Autodesk Inventor part; units mm, degrees
ref_plane "YZ Plane" through (0, 0, 0) normal (1, 0, 0) x (0, 1, 0)
ref_plane "XZ Plane" through (0, 0, 0) normal (0, 1, 0) x (-1, 0, 0)
ref_plane "XY Plane" through (0, 0, 0) normal (0, 0, 1) x (1, 0, 0)
sketch "Sketch1" plane through (0, 0, 0) normal (0, 0, 1) x (1, 0, 0)
  circle A0 centre (0, 0) radius 7
  circle A1 centre (52.2854, 37.1495) radius 7
  circle A2 centre (3.2487, 67.4218) radius 7
  circle A3 centre (73.2479, 48.3549) radius 2.15
  circle A4 centre (73.9366, 30.5749) radius 3.15 construction
  circle A5 centre (58.8599, 58.8007) radius 3.15 construction
  circle A6 centre (4.7755, 90.6548) radius 2.15
  circle A7 centre (-59.4554, -13.318) radius 2.15
  circle A8 centre (9.0171, -55.618) radius 2.15
  circle A9 centre (38.0853, -27.4589) radius 3.15 construction
  circle A10 centre (-27.4589, -38.0853) radius 3.5 construction
  line L0 (38.0853, -27.4589) -> (9.0171, -55.618) construction
  line L1 (9.0171, -55.618) -> (-27.4589, -38.0853) construction
  line L2 (9.0171, -55.618) -> (73.2479, 48.3549)
  line L3 (92.2333, 46.5881) -> (17.5545, -74.2973) construction
  line L4 (-27.4589, -38.0853) -> (-59.4554, -13.318) construction
  line L5 (-59.4554, -13.318) -> (-42.6755, 23.5008) construction
  line L6 (-59.4554, -13.318) -> (4.7755, 90.6548)
  line L7 (4.7755, 90.6548) -> (73.2479, 48.3549)
  line L8 (9.0171, -55.618) -> (-59.4554, -13.318)
  circle A11 centre (9.0171, -55.618) radius 6
  circle A12 centre (-59.4554, -13.318) radius 6
  circle A13 centre (4.7755, 90.6548) radius 6
  circle A14 centre (73.2479, 48.3549) radius 6
  point P0 (0, 0)
  point P1 (3.9125, -52.4646)
  point P2 (12.1704, -50.5134)
  point P3 (70.0945, 43.2504)
  point P4 (68.1434, 51.5083)
  point P5 (9.88, 87.5015)
  point P6 (1.6221, 85.5503)
  point P7 (-56.302, -8.2135)
  point P8 (-54.3509, -16.4714)
  point P9 (71.4188, 49.4849)
  point P10 (72.118, 46.5258)
  point P11 (3.6455, 88.8257)
  point P12 (6.6046, 89.5249)
  point P13 (-57.6263, -14.448)
  point P14 (-58.3254, -11.4889)
  point P15 (10.147, -53.7888)
  point P16 (7.1879, -54.488)
  dimension "d0" = 4.3
  dimension "d1" = 17.78
  dimension "d2" = 17.78
  dimension "d3" = 4.3
  dimension "d4" = 4.3
  dimension "d5" = 4.3
  dimension "d6" = 40.4622
  dimension "d7" = 12
  dimension "d8" = 12
  dimension "d9" = 12
  dimension "d10" = 12
extrude "Extrusion1" add sketch "Sketch1" along normal blind 3.175 contours A3 L7 A14 L2 | A3 L2 A14 L7 | A14 L2 A11 L8 A12 L6 A13 L7 | A13 L6 A6 L7 | L7 A6 L6 A13 | A11 L8 A8 L2 | L2 A8 L8 A11 | A12 L8 A7 L6 | L6 A7 L8 A12
fillet "Fillet1" radius 3.175 8 edges at (3.9125, -52.4646, 1.5875) (-54.3509, -16.4714, 1.5875) (-56.302, -8.2135, 1.5875) (1.6221, 85.5503, 1.5875) (9.88, 87.5015, 1.5875) (68.1434, 51.5083, 1.5875) (70.0945, 43.2504, 1.5875) (12.1704, -50.5134, 1.5875)
sketch "Sketch2" plane through (0, 0, 0) normal (0, 0, -1) x (-1, 0, 0)
  arc A0 (-13.742, -51.92) -> (-13.5412, -48.2946) centre (-16.2423, -49.9632) ccw
  line L0 (-13.5412, -48.2946) -> (-68.7238, 41.0315)
  arc A1 (-68.7238, 41.0315) -> (-72.0558, 42.4746) centre (-71.4249, 39.3629) ccw
  arc A2 (-69.55, 53.0799) -> (-72.0558, 42.4746) centre (-73.2479, 48.3549) ccw
  arc A3 (-69.55, 53.0799) -> (-65.9245, 52.8791) centre (-67.5932, 55.5802) ccw
  line L1 (-65.9245, 52.8791) -> (-12.0989, 86.1307)
  arc A4 (-12.0989, 86.1307) -> (-10.6559, 89.4627) centre (-13.7676, 88.8318) ccw
  arc A5 (-0.0505, 86.9569) -> (-10.6559, 89.4627) centre (-4.7755, 90.6548) ccw
  arc A6 (-0.0505, 86.9569) -> (-0.2513, 83.3315) centre (2.4498, 85.0001) ccw
  line L2 (-0.2513, 83.3315) -> (54.9312, -5.9946)
  arc A7 (54.9312, -5.9946) -> (58.2632, -7.4377) centre (57.6324, -4.326) ccw
  arc A8 (55.7575, -18.043) -> (58.2632, -7.4377) centre (59.4554, -13.318) ccw
  arc A9 (55.7575, -18.043) -> (52.132, -17.8422) centre (53.8007, -20.5433) ccw
  line L3 (52.132, -17.8422) -> (-1.6937, -51.0938)
  arc A10 (-1.6937, -51.0938) -> (-3.1367, -54.4258) centre (-0.025, -53.795) ccw
  arc A11 (-13.742, -51.92) -> (-3.1367, -54.4258) centre (-9.0171, -55.618) ccw
  circle A12 centre (-73.2479, 48.3549) radius 2.15
  circle A13 centre (0, 0) radius 7
  circle A14 centre (-52.2854, 37.1495) radius 7
  circle A15 centre (-3.2487, 67.4218) radius 7
  circle A16 centre (-4.7755, 90.6548) radius 2.15
  circle A17 centre (59.4554, -13.318) radius 2.15
  circle A18 centre (-9.0171, -55.618) radius 2.15
  line L4 (-50.3461, 20.9487) -> (-14.2871, -37.4213)
  arc A19 (-9.7416, -55.0509) -> (-9.2194, -45.6247) centre (-16.2423, -49.9632) ccw
  arc A20 (-9.7416, -55.0509) -> (-8.1154, -55.4352) centre (-9.0171, -55.618) ccw
  arc A21 (-4.3635, -46.772) -> (-8.1154, -55.4352) centre (-0.025, -53.795) ccw
  line L5 (0.8339, -43.5612) -> (42.6394, -17.7352)
  arc A22 (58.8884, -14.0425) -> (49.4621, -13.5204) centre (53.8007, -20.5433) ccw
  arc A23 (58.8884, -14.0425) -> (59.2726, -12.4164) centre (59.4554, -13.318) ccw
  arc A24 (50.6094, -8.6645) -> (59.2726, -12.4164) centre (57.6324, -4.326) ccw
  line L6 (46.6959, -2.3296) -> (9.6075, 57.7068)
  arc A25 (-4.051, 90.0878) -> (-4.5732, 80.6616) centre (2.4498, 85.0001) ccw
  arc A26 (-4.051, 90.0878) -> (-5.6771, 90.4721) centre (-4.7755, 90.6548) ccw
  arc A27 (-9.429, 81.8089) -> (-5.6771, 90.4721) centre (-13.7676, 88.8318) ccw
  line L7 (-11.3353, 80.6312) -> (-60.8723, 50.029)
  arc A28 (-72.6809, 49.0794) -> (-63.2547, 48.5572) centre (-67.5932, 55.5802) ccw
  arc A29 (-72.6809, 49.0794) -> (-73.0651, 47.4533) centre (-73.2479, 48.3549) ccw
  arc A30 (-64.402, 43.7014) -> (-73.0651, 47.4533) centre (-71.4249, 39.3629) ccw
  line L8 (-9.0171, -55.618) -> (0, 0) construction
  line L9 (0, 0) -> (59.4554, -13.318) construction
  line L10 (0, 0) -> (-3.2487, 67.4218) construction
  line L11 (-3.2487, 67.4218) -> (-4.7755, 90.6548) construction
  line L12 (0, 0) -> (-52.2854, 37.1495) construction
  line L13 (-52.2854, 37.1495) -> (-73.2479, 48.3549) construction
  line L14 (-52.2854, 37.1495) -> (-3.2487, 67.4218) construction
  line L15 (-4.7708, -13.5552) -> (-8.4519, -36.2607)
  line L16 (-11.5243, -55.2115) -> (-6.5098, -56.0245) construction
  line L17 (-3.9689, -40.352) -> (0.2437, -14.3682)
  line L18 (2.5073, -0.4065) -> (-2.5073, 0.4065) construction
  line L19 (-2.5073, 0.4065) -> (-6.5098, -56.0245) construction
  line L20 (-11.5243, -55.2115) -> (2.5073, -0.4065) construction
  line L21 (-39.2842, 31.0278) -> (-10.0588, 10.2628)
  line L22 (1.4712, 2.0706) -> (-1.4712, -2.0706) construction
  line L23 (-13.0012, 6.1217) -> (-42.2265, 26.8867)
  line L24 (-53.7566, 35.0789) -> (-50.8142, 39.2201) construction
  line L25 (-50.8142, 39.2201) -> (-1.4712, -2.0706) construction
  line L26 (1.4712, 2.0706) -> (-53.7566, 35.0789) construction
  line L27 (14.3572, -0.6131) -> (43.3008, -7.0964)
  line L28 (60.0106, -10.8395) -> (58.9002, -15.7966) construction
  line L29 (41.6647, -11.9359) -> (13.2468, -5.5702)
  line L30 (-0.5552, -2.4786) -> (0.5552, 2.4786) construction
  line L31 (0.5552, 2.4786) -> (58.9002, -15.7966) construction
  line L32 (60.0106, -10.8395) -> (-0.5552, -2.4786) construction
  line L33 (-3.2178, 14.0054) -> (-5.1051, 53.1719)
  line L34 (-5.7858, 67.2995) -> (-0.7117, 67.544) construction
  line L35 (-0.0309, 53.4164) -> (1.8563, 14.2499)
  line L36 (2.5371, 0.1222) -> (-2.5371, -0.1222) construction
  line L37 (-2.5371, -0.1222) -> (-0.7117, 67.544) construction
  line L38 (-5.7858, 67.2995) -> (2.5371, 0.1222) construction
  line L39 (-13.9498, 57.8305) -> (-38.9157, 42.4181)
  line L40 (-50.9511, 34.9882) -> (-53.6197, 39.3108) construction
  line L41 (-41.5843, 46.7407) -> (-16.6184, 62.1532)
  line L42 (-4.583, 69.5831) -> (-1.9145, 65.2604) construction
  line L43 (-1.9145, 65.2604) -> (-53.6197, 39.3108) construction
  line L44 (-50.9511, 34.9882) -> (-4.583, 69.5831) construction
  line L45 (-63.5617, 46.0573) -> (-60.7004, 44.5278)
  line L46 (-72.0505, 50.595) -> (-74.4453, 46.1149) construction
  line L47 (-74.4453, 46.1149) -> (-53.4828, 34.9094)
  line L48 (-53.4828, 34.9094) -> (-51.088, 39.3895) construction
  line L49 (-51.088, 39.3895) -> (-74.4453, 46.1149) construction
  line L50 (-72.0505, 50.595) -> (-53.4828, 34.9094) construction
  line L51 (-2.241, 90.8214) -> (-0.7142, 67.5883) construction
  line L52 (-0.7142, 67.5883) -> (-5.7833, 67.2552) construction
  line L53 (-6.7107, 81.3688) -> (-6.4984, 78.1383) construction
  line L54 (-7.31, 90.4883) -> (-2.241, 90.8214) construction
  line L55 (-2.241, 90.8214) -> (-5.7833, 67.2552) construction
  line L56 (-0.7142, 67.5883) -> (-7.31, 90.4883) construction
  arc A31 (-3.9689, -40.352) -> (0.8339, -43.5612) centre (-0.8348, -40.8601) ccw
  arc A32 (-14.2871, -37.4213) -> (-8.4519, -36.2607) centre (-11.586, -35.7526) ccw
  arc A33 (42.6394, -17.7352) -> (41.6647, -11.9359) centre (40.9707, -15.0341) ccw
  arc A34 (43.3008, -7.0964) -> (46.6959, -2.3296) centre (43.9948, -3.9982) ccw
  arc A35 (-5.1051, 53.1719) -> (-7.23, 56.0167) centre (-8.2764, 53.0191) ccw
  arc A36 (-8.499, 78.3012) -> (-6.7107, 81.3688) centre (-9.8789, 81.1606) ccw
  arc A37 (-8.499, 78.3012) -> (-15.1565, 65.3891) centre (-3.2487, 67.4218) ccw
  arc A38 (-10.4019, 57.6874) -> (-7.23, 56.0167) centre (-3.2487, 67.4218) ccw
  arc A39 (-10.4019, 57.6874) -> (-13.9498, 57.8305) centre (-12.282, 55.1289) ccw
  arc A40 (-16.6184, 62.1532) -> (-15.1565, 65.3891) centre (-18.2862, 64.8548) ccw
  arc A41 (-6.4984, 78.1383) -> (-11.3353, 80.6312) centre (-9.6666, 77.9301) ccw
  arc A42 (-40.5339, 34.3515) -> (-40.3776, 39.1822) centre (-52.2854, 37.1495) ccw
  arc A43 (-42.2265, 26.8867) -> (-45.7763, 26.9731) centre (-44.0655, 24.2985) ccw
  arc A44 (-45.1322, 46.8839) -> (-60.0296, 46.4206) centre (-52.2854, 37.1495) ccw
  arc A45 (-48.6108, 25.6419) -> (-45.7763, 26.9731) centre (-52.2854, 37.1495) ccw
  arc A46 (-48.6108, 25.6419) -> (-50.3461, 20.9487) centre (-47.645, 22.6174) ccw
  arc A47 (-45.1322, 46.8839) -> (-41.5843, 46.7407) centre (-43.2521, 49.4424) ccw
  arc A48 (-63.5617, 46.0573) -> (-60.0296, 46.4206) centre (-62.065, 48.8574) ccw
  arc A49 (-60.8723, 50.029) -> (-60.7004, 44.5278) centre (-59.2036, 47.3279) ccw
  arc A50 (-40.5339, 34.3515) -> (-39.2842, 31.0278) centre (-37.4452, 33.616) ccw
  arc A51 (-38.9157, 42.4181) -> (-40.3776, 39.1822) centre (-37.2479, 39.7164) ccw
  arc A52 (-5.0594, 10.9695) -> (-6.5091, 10.1764) centre (0, 0) ccw
  arc A53 (-11.7515, 2.798) -> (-6.2597, -10.3317) centre (0, 0) ccw
  arc A54 (2.6748, -11.7802) -> (9.9402, -6.8643) centre (0, 0) ccw
  arc A55 (11.9186, 1.9679) -> (3.9812, 11.4051) centre (0, 0) ccw
  arc A56 (-5.0594, 10.9695) -> (-3.2178, 14.0054) centre (-6.3891, 13.8526) ccw
  arc A57 (-10.0588, 10.2628) -> (-6.5091, 10.1764) centre (-8.2199, 12.851) ccw
  arc A58 (-11.7515, 2.798) -> (-13.0012, 6.1217) centre (-14.8401, 3.5334) ccw
  arc A59 (-4.7708, -13.5552) -> (-6.2597, -10.3317) centre (-7.9049, -13.0471) ccw
  arc A60 (2.6748, -11.7802) -> (0.2437, -14.3682) centre (3.3778, -14.8763) ccw
  arc A61 (13.2468, -5.5702) -> (9.9402, -6.8643) centre (12.5528, -8.6685) ccw
  arc A62 (11.9186, 1.9679) -> (14.3572, -0.6131) centre (15.0512, 2.4851) ccw
  arc A63 (1.8563, 14.2499) -> (3.9812, 11.4051) centre (5.0276, 14.4027) ccw
  arc A64 (1.8106, 56.4523) -> (4.7928, 58.4074) centre (-3.2487, 67.4218) ccw
  arc A65 (1.8106, 56.4523) -> (-0.0309, 53.4164) centre (3.1404, 53.5692) ccw
  arc A66 (9.6075, 57.7068) -> (4.7928, 58.4074) centre (6.9064, 56.0381) ccw
  point P0 (0, 0)
  point P1 (-4.5085, -27.809)
  point P2 (-26.1427, 18.5747)
  point P3 (29.7277, -6.659)
  point P4 (-1.6244, 33.7109)
  point P5 (-27.7671, 52.2856)
  point P6 (-62.7667, 42.7522)
  point P7 (-4.0121, 79.0383)
  point P8 (7.2726, 61.4864)
  point P9 (-52.9015, 25.0852)
  point P10 (-61.9209, 45.6857)
  point P11 (-7.0473, 79.7245)
  dimension "d14" = 5.08
  dimension "d15" = 5.08
  dimension "d16" = 5.08
  dimension "d17" = 5.08
  dimension "d18" = 5.08
  dimension "d19" = 5.08
  dimension "d20" = 5.08
  dimension "d21" = 5.08
  dimension "d22" = 3.175
  dimension "d25" = 3.175
  dimension "d26" = 3.175
  dimension "d27" = 3.175
  dimension "d29" = 3.175
  dimension "d30" = 3.175
  dimension "d31" = 3.175
  dimension "d32" = 3.175
  dimension "d34" = 3.175
  dimension "d35" = 5.08
  dimension "d36" = 3.175
  dimension "d37" = 3.175
extrude "Extrusion2" cut sketch "Sketch2" against normal blind 25.4 contours A46 A45 A43 L23 A58 A53 A59 L15 A32 L4 | A31 L17 A60 A54 A61 L29 A33 L5 | A34 L27 A62 A55 A63 L35 A65 A64 A66 L6 | A41 A36 A37 A40 L41 A47 A44 A48 A49 L7 | A50 A42 A51 L39 A39 A38 A35 L33 A56 A52 A57 L21
properties part number "Upper_Plate"
Can you work these out from the model? Positions are in its coordinate system, mm. Coordinates: 2 decimals unless noted, no trailing zeros. Order: outer loops, then holes, each group sorted by start corner. A loop starts at its lowest first (then second) coordinate and runs counter-clockwise, first axis right, second up. Notation, with made-up numbers: (59.5, 83.5) - (66.5, 83.5) arc R19 cw to (66.5, 100.5) - close; hole circle Ø10 at (7, -31). An arc over 180 degrees is marked (long way). Answer in a Markdown table with one row per item.
1. If I drill on line 1 along X through (y, z) = (51, 1.6); line 2 along X through (y, z) = (5, 2.4); line 3 along Y through (x, z) = (-30, 2.95), over which ranges is the centre line in solid material (lowest first)?
Reply:
| item | result |
|---|---|
| line 1 | x = -19.72 to -13.75, -0.09 to 5, 25.01 to 34.68, 59.3 to 78.63 |
| line 2 | x = -48.14 to -42.17, -11 to -4.9, 4.9 to 12.02, 40.49 to 46.46 |
| line 3 | y = -31.51 to -25.54, -9.32 to -4.12, 24.7 to 34.36 |
2. Suppose I cut it at A-A (y = -29.5). Please give me the cut outline in (x, z) (3 decimals).
Reply:
| item | result |
|---|---|
| outline | (-33.261, 0) - (-23.595, 0) - (-23.595, 3.175) - (-33.261, 3.175) - close; (2.21, 0) - (7.356, 0) - (7.356, 3.175) - (2.21, 3.175) - close; (19.181, 0) - (25.152, 0) - (25.152, 3.175) - (19.181, 3.175) - close |
3. If we mould it in two halves opening along X, with no side actions, what happens to faces 1 (the cylindrical face through (-46.55, -5.88, 1.57)), 2 (the cylindrical face through (3.233, 96.453, 1.565)), 3 (the cylindrical face through (-9.3, 7.71, 1.57)), 4 (the flat face through (1, 12, 0))? For each: pulls with the +X half, pulls with the -X half, needs draft (parallel to the pull), parting line crosses it, or undercut.
Reply:
| item | result |
|---|---|
| face 1 | undercut |
| face 2 | parting line crosses it |
| face 3 | undercut |
| face 4 | needs draft |
4. Suppose I cut it at D-D (z = 1.35). Give the number of separate pieces and of enclosed holes in the cut face, and give its area (3 significant figures).
Reply:
| item | result |
|---|---|
| separate pieces | 1 |
| enclosed holes | 12 |
| area | 4,080 mm^2 |
5. Suppose I cut it at C-C (y = 23.5). Please give me the cut outline in (x, z) (3 decimals).
Reply:
| item | result |
|---|---|
| outline | (-36.71, 0) - (-30.739, 0) - (-30.739, 3.175) - (-36.71, 3.175) - close; (-1.411, 0) - (3.675, 0) - (3.675, 3.175) - (-1.411, 3.175) - close; (28.689, 0) - (37.46, 0) - (37.46, 3.175) - (28.689, 3.175) - close; (50.695, 0) - (57.893, 0) - (57.893, 3.175) - (50.695, 3.175) - close |
6. Suppose I cut it at B-B (x = -19.5). Please give me the cut outline in (y, z) (3 decimals), and give its area (3 significant figures).
Reply:
| item | result |
|---|---|
| outline | (-38.001, 0) - (-32.03, 0) - (-32.03, 3.175) - (-38.001, 3.175) - close; (-6.971, 0) - (-1.765, 0) - (-1.765, 3.175) - (-6.971, 3.175) - close; (41.693, 0) - (51.359, 0) - (51.359, 3.175) - (41.693, 3.175) - close |
| area | 66.2 mm^2 |
7. For pin 1 (1 mm diameter, centred on x = 46, z = 1.5, fed in from -Y), with a flat end and sliding along its axis, tell me the tip position at first contact or that it passes through.
Reply:
| item | result |
|---|---|
| pin 1 | stops at y = 3.44 |
